The drawing under review shows one solid part. Ordinate dimensions are in mm from its lowest x, y, z. A direction names the side the tool comes from. Round coordinates to 2 decimals unless told otherwise and drop trailing zeros. Order: outer loops, then holes, each group sorted by start corner. A loop starts at its lowest first (then second) coordinate and runs counter-clockwise, first axis right, second up. Notation, with made-up numbers: (53.25, 3.5) -> (63.25, 3.5) arc R8 cw to (63.25, 13.5) -> close; hole circle Ø4 at (-6, 70.25). An arc over 180 degrees is marked (long way). Use a Markdown table: item, result. Add a question column.
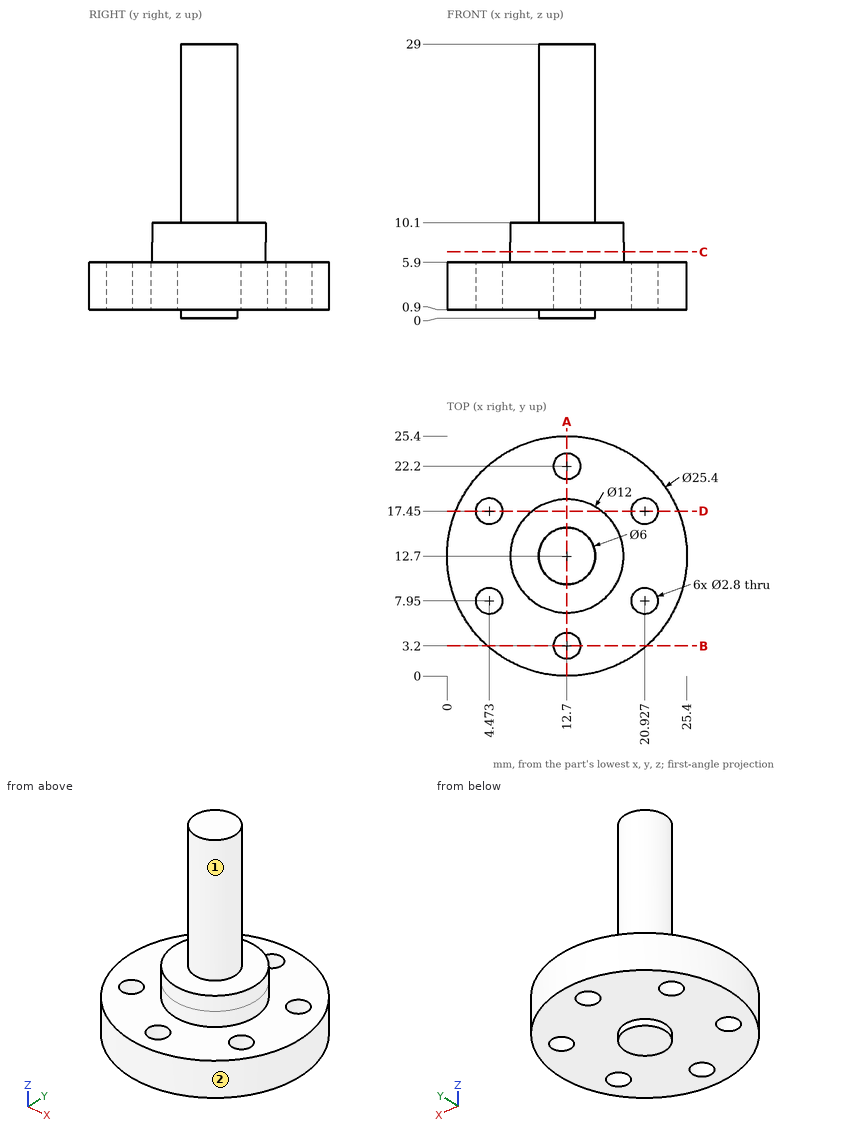
Q1. To check wall thickness, follow line 1 along Y through (x, z) = (20.5, 5.5); line 2 along Y through (x, z) = (12.5, 2.25); line 3 along Z through (x, y) = (6.25, 3). State the ranges of each line that lie inside material, in increasing order.
Q2. Add section C-C, the plane z = 7. Give the boundary of the cut face in (x, y).
Q3. For pin 1 (6 mm diameter, centred on x = 4.5, y = 8.5, fed in from -Z); pin 2 (2 mm diameter, centred on x = 10.5, y = 21, fed in from +Z); pin 3 (4 mm diameter, centred on y = 13, z = 9, fed in from +X), all flat-tipped, find the tip position at first contact; note any pin that passes through.
Q4. Add section D-D, the plane y = 17.45. Give the boundary of the cut face in (x, z), then the cut area to 3 significant figures.
Q5. Add section A-A, the plane x = 12.7. Give the boundary of the cut face in (y, z).
Q6. Add section B-B, the plane y = 3.2. Give the boundary of the cut face in (x, z).
Q7. For the marked faces 1 and 2, list the 3-axis set-ups (+Z, -Z, +X, -X, +Y, -Y) from which the entire face can be reached by the end or side of a thin tool; tool diameter is ignored.
Return value:
| question | item | result |
|---|---|---|
| 1 | line 1 | 2.68 to 6.62, 9.28 to 16.12, 18.78 to 22.72 |
| 1 | line 2 | 0 to 1.81, 4.59 to 20.81, 23.59 to 25.4 |
| 1 | line 3 | 0.9 to 5.9 |
| 2 | outline | circle Ø12 at (12.7, 12.7) |
| 3 | pin 1 | z = 0.9 |
| 3 | pin 2 | z = 5.9 |
| 3 | pin 3 | x = 18.7 |
| 4 | outline | (0.92, 0.9) -> (3.07, 0.9) -> (3.07, 5.9) -> (0.92, 5.9) -> close; (5.87, 0.9) -> (19.53, 0.9) -> (19.53, 5.9) -> (16.37, 5.9) -> (16.37, 10.1) -> (9.03, 10.1) -> (9.03, 5.9) -> (5.87, 5.9) -> close; (22.33, 0.9) -> (24.48, 0.9) -> (24.48, 5.9) -> (22.33, 5.9) -> close |
| 4 | area | 121 mm² |
| 5 | outline | (0, 0.9) -> (1.8, 0.9) -> (1.8, 5.9) -> (0, 5.9) -> close; (4.6, 0.9) -> (9.7, 0.9) -> (9.7, 0) -> (15.7, 0) -> (15.7, 0.9) -> (20.8, 0.9) -> (20.8, 5.9) -> (18.7, 5.9) -> (18.7, 10.1) -> (15.7, 10.1) -> (15.7, 29) -> (9.7, 29) -> (9.7, 10.1) -> (6.7, 10.1) -> (6.7, 5.9) -> (4.6, 5.9) -> close; (23.6, 0.9) -> (25.4, 0.9) -> (25.4, 5.9) -> (23.6, 5.9) -> close |
| 6 | outline | (4.27, 0.9) -> (11.3, 0.9) -> (11.3, 5.9) -> (4.27, 5.9) -> close; (14.1, 0.9) -> (21.13, 0.9) -> (21.13, 5.9) -> (14.1, 5.9) -> close |
| 7 | face 1 | +Z |
| 7 | face 2 | +Z, -Z |
